Check sheet for the modelled part. Datum: model origin and axes. Units: mm. Round coordinates to 2 decimals unless told otherwise and drop trailing zeros. Loops run counter-clockwise (first coordinate to the right, second up) from the corner with the lowest first, then second, coordinate; pieces in that order, holes last. Notation, with made-up numbers: (21.5, -11) - (55.5, -11) arc R21 cw to (55.5, -4) - close; hole circle Ø10 at (6, 16.5). An arc over 180 degrees is marked (long way). Put each result on its own line as item: value. Start each with the question number.
Item 1: Draft check along Z on faces 1 (the cylindrical face through (202.7, -6.26, 32.63)), 2 (the flat face through (106, -6, 0)), 3 (the flat face through (125, -12.7, 39)). Enter one of: pulls with the +Z half, pulls with the -Z half, needs draft (parallel to the pull), parting line crosses it, or undercut.
Item 2: Gauge pin test, flat ends, axial feed: pin 1 Ø4 at (x, y) = (131.5, -7) entering from -Z; pin 2 Ø6 at (y, z) = (-7.5, 46.5) entering from +X. Record the tip position at first contact, or that the pin passes through.
Item 3: Material ranges on line 1 along Z through (x, y) = (215.9, -2.5); line 2 along X through (y, z) = (-4.75, 37); line 3 along X through (y, z) = (-7.5, 30), recorded low to high.
Item 4: Section check D-D, the plane z = 60.5. Record the cut outline in (x, y).
Item 5: Section check A-A, the plane z = 31. Record the cut outline in (x, y), and give its area (3 significant figures).
Item 6: Section check C-C, the plane x = 224. Record the cut outline in (y, z), and give its area (3 significant figures).
Item 7: Section check B-B, the plane y = -7.75. Record the cut outline in (x, z) (1 decimal).
from build123d import *

# Parameters (mm, degrees)
F1_DEPTH = 12.7


with BuildPart() as f1:
    # F0 (on Front) → F1 (new body)
    with BuildSketch(Plane.XZ):
        with BuildLine():
            Line((0, 38.1), (0, 0))
            Line((0, 0), (215.9, 0))
            ThreePointArc((215.9, 0), (242.840768, 11.159232), (254, 38.1))
            ThreePointArc((254, 38.1), (242.840768, 65.040768), (215.9, 76.2))
            Line((215.9, 76.2), (0, 76.2))
            Line((0, 76.2), (0, 38.1))
        make_face()
        with BuildLine():
            ThreePointArc((230.1875, 38.1), (215.9, 23.8125), (201.6125, 38.1))
            ThreePointArc((201.6125, 38.1), (215.9, 52.3875), (230.1875, 38.1))
        make_face(mode=Mode.SUBTRACT)
    extrude(amount=F1_DEPTH)


solid = f1.part
Check result:
1. face 1: undercut
1. face 2: pulls with the -Z half
1. face 3: needs draft
2. pin 1: z = 0
2. pin 2: x = 253.62
3. line 1: 0 to 23.81, 52.39 to 76.2
3. line 2: 0 to 201.65, 230.15 to 253.98
3. line 3: 0 to 204.13, 227.67 to 253.13
4. outline: (0, -12.7) - (246.72, -12.7) - (246.72, 0) - (0, 0) - close
5. outline: (0, -12.7) - (203.5, -12.7) - (203.5, 0) - (0, 0) - close; (228.3, -12.7) - (253.33, -12.7) - (253.33, 0) - (228.3, 0) - close
5. area: 2,900 mm²
6. outline: (-12.7, 0.87) - (0, 0.87) - (0, 26.33) - (-12.7, 26.33) - close; (-12.7, 49.87) - (0, 49.87) - (0, 75.33) - (-12.7, 75.33) - close
6. area: 647 mm²
7. outline: (0, 0) - (215.9, 0) arc R38.1 ccw to (254, 38.1) arc R38.1 ccw to (215.9, 76.2) - (0, 76.2) - close; hole circle Ø28.6 at (215.9, 38.1)
